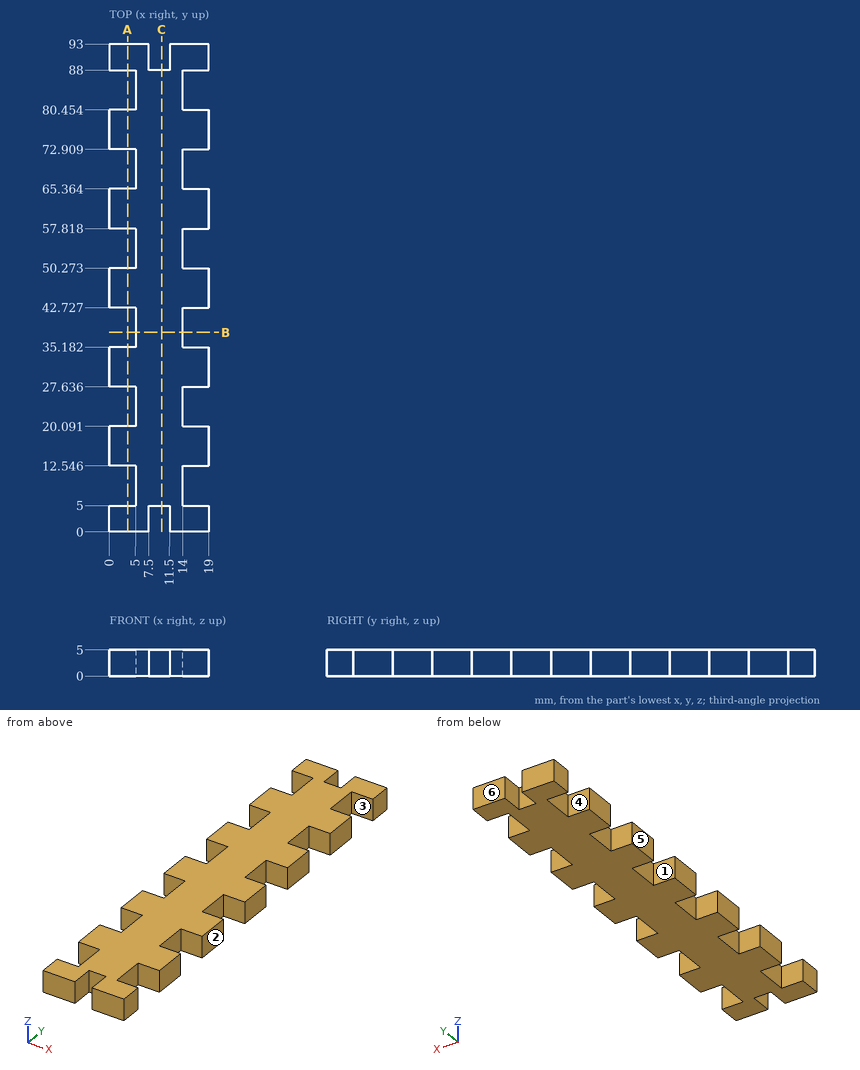
For this review, use the dimensioned drawing (mm, ordinates from the lowest corner) and the shaded views. A direction names the side the tool comes from. Round coordinates to 2 decimals unless told otherwise and drop trailing zeros. Order: outer loops, then holes, each group sorted by start corner. A loop starts at its lowest first (then second) coordinate and runs counter-clockwise, first axis right, second up. Notation, with made-up numbers: (75.25, 79) -> (110.25, 79) arc R19 cw to (110.25, 105) -> close; hole circle Ø3 at (23, 21.5). An arc over 180 degrees is marked (long way). Put each result on its own line as item: value.
Q1. For probe 1 along X at (y, z) = (54, 4.4); probe 2 along Y at (x, z) = (7.75, 3.6), list the stretches that pass through material, from the lowest coordinate up. Write a range as [from, to].
Check result:
probe 1: [5, 14]
probe 2: [5, 88]
Q2. Mouldability with a two-part tool opening along Y and no side actions: class the marked faces 4, 5 and 6 as pulls with the +Y half, pulls with the -Y half, needs draft (parallel to the pull), parting line crosses it, or undercut.
Check result:
face 4: undercut
face 5: needs draft
face 6: pulls with the +Y half
Q3. Insertion check: pin 1 Ø2 at (x, z) = (9, 2.5) entering from -Y; pin 2 Ø2.5 at (y, z) = (70.5, 2.5) entering from +X; pin 3 Ø1.5 at (x, z) = (16.5, 1.5) entering from -Y; pin 4 Ø2.5 at (y, z) = (39.5, 2.5) entering from -X. Each pin has a flat end and moves straight along its axis. Give the tip position at first contact, or say it passes through.
Check result:
pin 1: y = 5
pin 2: x = 14
pin 3: y = 0
pin 4: x = 5
Q4. Add section B-B on y = 38. Write out the cut boundary in (x, z), plus the area to 3 significant figures.
Check result:
outline: (5, 0) -> (14, 0) -> (14, 5) -> (5, 5) -> close
area: 45.0 mm2
Q5. Add section C-C on x = 10. Write out the cut boundary in (y, z), plus the area to 3 significant figures.
Check result:
outline: (5, 0) -> (88, 0) -> (88, 5) -> (5, 5) -> close
area: 415 mm2
Q6. Machinability: for the marked faces 1, 2 and 3, which of the approach directions +Z, -Z, +X, -X, +Y, -Y give a long, thin tool a straight path to every point of the face, cutting with its end or side? Answer none if there is none.
Check result:
face 1: +Z, -Z, -X
face 2: +Z, -Z, +X, +Y, -Y
face 3: +Z, -Z, +X
Q7. Add section A-A on x = 3.5. Write out the cut boundary in (y, z) (1 decimal).
Check result:
outline: (0, 0) -> (5, 0) -> (5, 5) -> (0, 5) -> close; (12.5, 0) -> (20.1, 0) -> (20.1, 5) -> (12.5, 5) -> close; (27.6, 0) -> (35.2, 0) -> (35.2, 5) -> (27.6, 5) -> close; (42.7, 0) -> (50.3, 0) -> (50.3, 5) -> (42.7, 5) -> close; (57.8, 0) -> (65.4, 0) -> (65.4, 5) -> (57.8, 5) -> close; (72.9, 0) -> (80.5, 0) -> (80.5, 5) -> (72.9, 5) -> close; (88, 0) -> (93, 0) -> (93, 5) -> (88, 5) -> close
